Read the model definition and answer for the solid it produces. Units are mm, in the model's axes. A direction names the side the tool comes from. Coordinates: 2 decimals unless noted, no trailing zeros. Loops run counter-clockwise (first coordinate to the right, second up) from the corner with the lowest first, then second, coordinate; pieces in that order, holes last. Notation, with made-up numbers: (-19, -17.5) -> (2, -17.5) arc R5 cw to (2, -9.5) -> close; hole circle Ø5 at (42, 18.25). An arc over 180 degrees is marked (long way). Answer in a Markdown table with one row per item.
```python
from build123d import *

# Parameters (mm, degrees)
SKETCH015_W     = 157.6
SKETCH015_H     = 280
SKETCH015_R     = 1.55
PAD007_DEPTH    = 4
SKETCH016_R     = 18.25
SKETCH016_W     = 52
SKETCH016_H     = 79.3
POCKET008_DEPTH = 10
SKETCH017_R     = 20.5
SKETCH017_W     = 56.5
SKETCH017_H     = 86.5
POCKET009_DEPTH = 2
PAD008_DEPTH    = 2
SKETCH019_R     = 1.55
POCKET010_DEPTH = 9


with BuildPart() as part:
    # Sketch015 (on ShapeBinder) → Pad007 (new body)
    with BuildSketch(Plane(origin=(0, 0, 46), x_dir=(0, -1, 0), z_dir=(0, 0, 1))):
        with Locations((-72.5, 140)):
            Rectangle(SKETCH015_W, SKETCH015_H)
        with Locations((-146.8, 275.5)):
            Circle(SKETCH015_R, mode=Mode.SUBTRACT)
        with Locations((1.8, 275.5)):
            Circle(SKETCH015_R, mode=Mode.SUBTRACT)
        with Locations((-146.8, 4.5)):
            Circle(SKETCH015_R, mode=Mode.SUBTRACT)
        with Locations((1.8, 4.5)):
            Circle(SKETCH015_R, mode=Mode.SUBTRACT)
    extrude(amount=PAD007_DEPTH)

    # Sketch016 (on Face10 of Pad007) → Pocket008 (cut)
    with BuildSketch(Plane(origin=(0, 0, 50), x_dir=(0, -1, 0), z_dir=(0, 0, 1))):
        with Locations((-117.7, 50)):
            Circle(SKETCH016_R)
        with Locations((-117.7, 230)):
            Circle(SKETCH016_R)
        with Locations((-44, 109.65)):
            Rectangle(SKETCH016_W, SKETCH016_H)
    extrude(amount=-POCKET008_DEPTH, mode=Mode.SUBTRACT)

    # Sketch017 (on Face4 of Pocket008) → Pocket009 (cut)
    with BuildSketch(Plane.YX.offset(-46)):
        with Locations((117.7, 230)):
            Circle(SKETCH017_R)
        with Locations((117.7, 50)):
            Circle(SKETCH017_R)
        with Locations((43.85, 111.75)):
            Rectangle(SKETCH017_W, SKETCH017_H)
    extrude(amount=-POCKET009_DEPTH, mode=Mode.SUBTRACT)

    # Sketch018 (on Face5 of Pocket009) → Pad008 (join)
    with BuildSketch(Plane(origin=(0, 0, 50), x_dir=(0, -1, 0), z_dir=(0, 0, 1))):
        Polygon((-142.58252, 252.331589), (-142.58252, 256.331589), (-92.58252, 234.331589), (-92.58252, 230.331589), align=None)
        Polygon((-142.58252, 243.331589), (-142.58252, 247.331589), (-92.58252, 225.331589), (-92.58252, 221.331589), align=None)
        Polygon((-142.58252, 234.331589), (-142.58252, 238.331589), (-92.58252, 216.331589), (-92.58252, 212.331589), align=None)
        Polygon((-142.58252, 225.331589), (-142.58252, 229.331589), (-92.58252, 207.331589), (-92.58252, 203.331589), align=None)
        Polygon((-142.313179, 71.876823), (-142.313179, 75.876823), (-92.313179, 53.876823), (-92.313179, 49.876823), align=None)
        Polygon((-142.313179, 62.876823), (-142.313179, 66.876823), (-92.313179, 44.876823), (-92.313179, 40.876823), align=None)
        Polygon((-142.313179, 53.876823), (-142.313179, 57.876823), (-92.313179, 35.876823), (-92.313179, 31.876823), align=None)
        Polygon((-142.313179, 44.876823), (-142.313179, 48.876823), (-92.313179, 26.876823), (-92.313179, 22.876823), align=None)
    extrude(amount=-PAD008_DEPTH)

    # Sketch019 (on Face4 of Pad008) → Pocket010 (cut)
    with BuildSketch(Plane.YX.offset(-46)):
        with Locations((11.6, 159.5)):
            Circle(SKETCH019_R)
        with Locations((76.6, 159.5)):
            Circle(SKETCH019_R)
        with Locations((76.6, 64.5)):
            Circle(SKETCH019_R)
        with Locations((11.6, 64.5)):
            Circle(SKETCH019_R)
    extrude(amount=-POCKET010_DEPTH, mode=Mode.SUBTRACT)


solid = part.part
```
1. The mould has two halves that part along Y. Classify faces 1 (the flat face through (142, 74, 50)), 2 (the cylindrical face through (247.3, 128.7, 47)): pulls with the +Y half, pulls with the -Y half, needs draft (parallel to the pull), parting line crosses it, or undercut.
A:
| item | result |
|---|---|
| face 1 | needs draft |
| face 2 | undercut |
2. A cutting plane is placed at C-C on y = 25. Give the vertices of the cut face in (x, z), and give its area (3 significant figures).
A:
| item | result |
|---|---|
| outline | (0, 46) -> (68.5, 46) -> (68.5, 48) -> (70, 48) -> (70, 50) -> (0, 50) -> close; (149.3, 48) -> (155, 48) -> (155, 46) -> (280, 46) -> (280, 50) -> (149.3, 50) -> close |
| area | 788 mm2 |
3. A cutting plane is placed at B-B on x = 139.5. Give the vertices of the cut face in (y, z).
A:
| item | result |
|---|---|
| outline | (-6.3, 46) -> (15.6, 46) -> (15.6, 48) -> (18, 48) -> (18, 50) -> (-6.3, 50) -> close; (70, 48) -> (72.1, 48) -> (72.1, 46) -> (151.3, 46) -> (151.3, 50) -> (70, 50) -> close |
4. A tool of negligible diameter and unlimited length cuts with its end or side. For faces 3 (the flat face through (220.35, 122.17, 49.01)), 4 (the cylindrical face through (42.148, 136.637, 46.986)), from which of +Z, -Z, +X, -X, +Y, -Y can it reach the whole face along a straight path? Write none if from no direction.
A:
| item | result |
|---|---|
| face 3 | +Z, -Z |
| face 4 | -Z |
5. Given pin 1 Ø12.5 at (x, y) = (45, 122) entering from -Z, flat-ended and moving along its own axis, determine where the tip first touches the part or whether it passes through.
A:
| item | result |
|---|---|
| pin 1 | stops at z = 48 |
6. Find the intervals of material crossed by probe 1 along X at (y, z) = (11.6, 48.95); probe 2 along Y at (x, z) = (275.5, 47.35); probe 3 along X at (y, z) = (-1.8, 49.15), in increasing order.
A:
| item | result |
|---|---|
| probe 1 | x = 0 to 62.95, 66.05 to 157.95, 161.05 to 280 |
| probe 2 | y = -6.3 to -3.35, -0.25 to 145.25, 148.35 to 151.3 |
| probe 3 | x = 0 to 2.95, 6.05 to 273.95, 277.05 to 280 |
7. A cutting plane is placed at A-A on z = 47.3. Count the separate pieces of the cut face and the enclosed holes in it, and give its area (3 significant figures).
A:
| item | result |
|---|---|
| separate pieces | 1 |
| enclosed holes | 11 |
| area | 36,500 mm2 |
